Check sheet for the modelled part. Datum: model origin and axes. Units: mm. A direction names the side the tool comes from. Round coordinates to 2 decimals unless told otherwise and drop trailing zeros. Loops run counter-clockwise (first coordinate to the right, second up) from the corner with the lowest first, then second, coordinate; pieces in that order, holes last. Notation, with made-up numbers: (-6, 55) -> (14, 55) arc R31 cw to (14, 92) -> close; hole circle Ø9 at (10, -35.75). An arc over 180 degrees is marked (long way). One line per item, written item: value. Start each with the question number.
1. Set-up check for faces 4 (the face through (8, 2.8, 8)), 5 (the face through (0, 6, 0)), 6 (the face through (10.035, 0.923, 2.426)): record each of +Z, -Z, +X, -X, +Y, -Y from which the full face is reachable in a straight line by a thin tool's end or side.
2. Cross-section at C-C on x = 0. Record the cut outline in (y, z).
3. Go/stop test with a flat-tipped pin: pin 1 (2.5 mm diameter, centred on y = 0, z = 4.2, fed in from +X). Record where the tip stops, or that it passes through.
4. Material ranges on L1, parallel to Y at x = 10.4, z = 4.2; L2, parallel to Z at x = 10.2, y = 0; L3, parallel to X at y = -0.5, z = 9, recorded low to high.
5. Cross-section at A-A on y = 0. Record the cut outline in (x, z), then the cut area to 3 significant figures.
6. Release check for a two-part mould opening along X. For faces 1 (the face through (-12.5, 0, 5)), 2 (the face through (-1.19, -5.37, 4.93)), 3 (the face through (0, 12.5, 5)) record: +X half, -X half, draft (parallel to the pull), parting line (faces both ways), or undercut.
7. Cross-section at D-D on z = 1.5. Record the cut outline in (x, y), then the cut area to 3 significant figures.
8. Cross-section at B-B on z = 8.25. Record the cut outline in (x, y).
from build123d import *

# Parameters (mm, degrees)
SKETCH_W        = 25
SKETCH_H        = 25
SKETCH_R        = 5.5
PAD_DEPTH       = 10
SKETCH001_R     = 2
POCKET_DEPTH    = 5
SKETCH002_W     = 2.5
SKETCH002_H     = 5.6
POCKET001_DEPTH = 5


with BuildPart() as part:
    # Sketch → Pad (new body)
    with BuildSketch(Plane.XY):
        Rectangle(SKETCH_W, SKETCH_H)
        Circle(SKETCH_R, mode=Mode.SUBTRACT)
    extrude(amount=PAD_DEPTH)

    # Sketch001 (on Face1 of Pad) → Pocket (cut)
    with BuildSketch(Plane.YZ.offset(12.5)):
        with Locations((0, 4.2)):
            Circle(SKETCH001_R)
    extrude(amount=-POCKET_DEPTH, mode=Mode.SUBTRACT)

    # Sketch002 (on Face4 of Pocket) → Pocket001 (cut)
    with BuildSketch(Plane.XY.offset(10)):
        with Locations((8.25, 0)):
            Rectangle(SKETCH002_W, SKETCH002_H)
    extrude(amount=-POCKET001_DEPTH, mode=Mode.SUBTRACT)


solid = part.part
Taken from the geometry:
1. face 4: +Z
1. face 5: -Z, +X, -X, +Y, -Y
1. face 6: +X
2. outline: (-12.5, 0) -> (-5.5, 0) -> (-5.5, 10) -> (-12.5, 10) -> close; (5.5, 0) -> (12.5, 0) -> (12.5, 10) -> (5.5, 10) -> close
3. pin 1: stops at x = 7.5
4. L1: y = -12.5 to -2, 2 to 12.5
4. L2: z = 0 to 2.2, 6.2 to 10
4. L3: x = -12.5 to -5.48, 5.48 to 7, 9.5 to 12.5
5. outline: (-12.5, 0) -> (-5.5, 0) -> (-5.5, 10) -> (-12.5, 10) -> close; (5.5, 0) -> (12.5, 0) -> (12.5, 2.2) -> (7.5, 2.2) -> (7.5, 5) -> (7, 5) -> (7, 10) -> (5.5, 10) -> close; (9.5, 6.2) -> (12.5, 6.2) -> (12.5, 10) -> (9.5, 10) -> close
5. area: 110 mm2
6. face 1: -X half
6. face 2: undercut
6. face 3: draft
7. outline: (-12.5, -12.5) -> (12.5, -12.5) -> (12.5, 12.5) -> (-12.5, 12.5) -> close; hole circle Ø11 at (0, 0)
7. area: 530 mm2
8. outline: (-12.5, -12.5) -> (12.5, -12.5) -> (12.5, 12.5) -> (-12.5, 12.5) -> close; hole circle Ø11 at (0, 0); hole (7, -2.8) -> (9.5, -2.8) -> (9.5, 2.8) -> (7, 2.8) -> close
